from build123d import *

# Parameters (mm, degrees)
SKETCH1_R           = 45
BOSS_EXTRUDE1_DEPTH = 150
SKETCH2_R           = 30
BOSS_EXTRUDE2_DEPTH = 50
SKETCH3_R           = 15
BOSS_EXTRUDE3_DEPTH = 35


with BuildPart() as part:
    # Sketch1 → Boss-Extrude1 (new, symmetric)
    with BuildSketch(Plane.XY):
        Circle(SKETCH1_R)
    extrude(amount=BOSS_EXTRUDE1_DEPTH, both=True)

    # Sketch2 → Boss-Extrude2 (add)
    with BuildSketch(Plane.XY.offset(150)):
        Circle(SKETCH2_R)
    boss_extrude2 = extrude(amount=BOSS_EXTRUDE2_DEPTH)

    # Sketch3 → Boss-Extrude3 (add)
    with BuildSketch(Plane.XY.offset(200)):
        Circle(SKETCH3_R)
    boss_extrude3 = extrude(amount=BOSS_EXTRUDE3_DEPTH)

    # Mirror2: Boss-Extrude2, Boss-Extrude3 across plane
    add(boss_extrude2.mirror(Plane.XY))
    add(boss_extrude3.mirror(Plane.XY))


solid = part.part
Can you work these out from the model? Positions are in its coordinate system, mm. A direction names the side the tool comes from. Coordinates: 2 decimals unless noted, no trailing zeros. Order: outer loops, then holes, each group sorted by start corner. A loop starts at its lowest first (then second) coordinate and runs counter-clockwise, first axis right, second up. Notation, with made-up numbers: (38.25, 53) - (90.25, 53) arc R26 ccw to (90.25, 72) - close; hole circle Ø6 at (-24.75, 36). An arc over 180 degrees is marked (long way). Answer as a JSON object with one key per item and string values. Group by question number.
Q1. On a 3-axis mill with a long thin cutter (end or side, diameter ignored), from which of +Z, -Z, +X, -X, +Y, -Y can I reach the whole of each face in a straight line? I mean faces 1 (the face through (0, 0, 235)), 2 (the face through (-14.985, 0.66, -217.255)), 3 (the face through (29, -9, 150)). Say none if no direction works.
Q2. Will these pins go through, and if not, where does the flat tip stop? P1, Ø5, axis at y = -2.5, z = 15, coming from the -X side; P2, Ø4, axis at x = -3, z = 132.5, coming from the -Y side; P3, Ø6, axis at x = -10, y = -26.5, coming from the -Z side; P4, Ø3, axis at y = 16.5, z = -85, coming from the -X side.
Q3. Imagine slicing it at A-A (y = 0). Please give me the cut outline in (x, z).
Q4. I need wall thicknesses on line 1 (Z direction, x = 31, y = 12.5); line 2 (Z direction, x = 24, y = 11); line 3 (Y direction, x = 0.5, z = -30). Which ranges of each line are inside material? Lowest first, please. Write a range as from..to.
Q5. Imagine slicing it at D-D (x = -24). Please give me the cut outline in (y, z), and give its area (3 significant figures).
Q6. Imagine slicing it at B-B (x = 1). Please give me the cut outline in (y, z).
Q7. Imagine slicing it at C-C (z = -49). Please give me the cut outline in (x, y), and give its area (3 significant figures).
Determined:
{
 "1": {"face 1": "+Z, +X, -X, +Y, -Y", "face 2": "-Z", "face 3": "+Z"},
 "2": {"P1": "stops at x = -45", "P2": "stops at y = -44.99", "P3": "stops at z = -200", "P4": "stops at x = -42.43"},
 "3": {"outline": "(-45, -150) - (-30, -150) - (-30, -200) - (-15, -200) - (-15, -235) - (15, -235) - (15, -200) - (30, -200) - (30, -150) - (45, -150) - (45, 150) - (30, 150) - (30, 200) - (15, 200) - (15, 235) - (-15, 235) - (-15, 200) - (-30, 200) - (-30, 150) - (-45, 150) - close"},
 "4": {"line 1": "z = -150..150", "line 2": "z = -200..200", "line 3": "y = -45..45"},
 "5": {"outline": "(-38.07, -150) - (-18, -150) - (-18, -200) - (18, -200) - (18, -150) - (38.07, -150) - (38.07, 150) - (18, 150) - (18, 200) - (-18, 200) - (-18, 150) - (-38.07, 150) - close", "area": "26,400 mm2"},
 "6": {"outline": "(-44.99, -150) - (-29.98, -150) - (-29.98, -200) - (-14.97, -200) - (-14.97, -235) - (14.97, -235) - (14.97, -200) - (29.98, -200) - (29.98, -150) - (44.99, -150) - (44.99, 150) - (29.98, 150) - (29.98, 200) - (14.97, 200) - (14.97, 235) - (-14.97, 235) - (-14.97, 200) - (-29.98, 200) - (-29.98, 150) - (-44.99, 150) - close"},
 "7": {"outline": "circle Ø90 at (0, 0)", "area": "6,360 mm2"}
}
